The model under review builds one solid part; all positions refer to its coordinate system, in mm. A direction names the side the tool comes from. Round coordinates to 2 decimals unless told otherwise and drop trailing zeros. Order: outer loops, then holes, each group sorted by start corner. A loop starts at its lowest first (then second) coordinate and runs counter-clockwise, first axis right, second up. Notation, with made-up numbers: M -29,69.25 L 0,69.25 A13 ccw 0,76.25 Z; hole C 44,7 d4. An arc over 180 degrees is marked long. Answer as a JSON object with one key per item and string values. Group by question number.
1) Consider section D-D, the plane y = -8.25. Write out the cut boundary in (x, z), then the cut area to 3 significant figures.
2) To check wall thickness, follow line 1 (Y direction, x = 19, z = 32); line 2 (X direction, y = -21.75, z = -34.5); line 3 (Z direction, x = 38, y = -12.25). State the ranges of each line that lie inside material, in increasing order.
3) Consider section B-B, the plane y = -17. Write out the cut boundary in (x, z), then the cut area to 3 significant figures.
4) Consider section C-C, the plane z = 25.5. Write out the cut boundary in (x, y).
5) Consider section A-A, the plane x = -28.5. Write out the cut boundary in (y, z), then the cut area to 3 significant figures.
6) Insertion check: pin 1 Ø12 at (x, z) = (-23, -0.5) entering from -Y; pin 2 Ø10 at (x, z) = (-68, 15.5) entering from +Y; pin 3 Ø1.3 at (x, y) = (-32, -26.5) entering from -Z. Each pin has a flat end and moves straight along its axis. Give the tip position at first contact, or say it passes through.
7) For faces 1 (the cylindrical face through (42.55, -2.02, 8.81)), 2 (the flat face through (-30, -28, 32.298)), 3 (the cylindrical face through (-65.101, -22.062, 4.926)), 4 (the flat face through (-30, -28, 21.446)), 5 (the flat face through (-21.4, -28, 27)), list the 3-axis set-ups (+Z, -Z, +X, -X, +Y, -Y) from which the entire face can be reached by the end or side of a thin tool; tool diameter is ignored.
```python
from build123d import *

# Parameters (mm, degrees)
F0_W      = 68.2077519596
F0_H      = 90.4731266201
F1_DEPTH  = 25.4
F2_R      = 10.4447594079
F3_DEPTH  = 30.0825480372
F4_R      = 9.9602632564
F5_DEPTH  = 25.4
F6_DEPTH  = 14.6486386657
F7_DEPTH  = 77.0113542676
F8_DEPTH  = 7.2514917701
F9_DEPTH  = 2.6144357398
F10_W     = 17.0795619488
F10_H     = 10.8526591212
F11_DEPTH = 4.2919376865


with BuildPart() as f1:
    # F0 (on Front) → F1 (new body)
    with BuildSketch(Plane.XZ):
        with Locations((-11.2533476204, -0.3619696945)):
            Rectangle(F0_W, F0_H)
    extrude(amount=F1_DEPTH)

    # F2 (on face) → F3 (join)
    with BuildSketch(Plane.YZ.offset(22.8505283594)):
        with Locations((-11.9834244251, 5.6728608906)):
            Circle(F2_R)
    extrude(amount=F3_DEPTH)

    # F4 (on face) → F5 (join)
    with BuildSketch(Plane(origin=(-45.3572236001, 0, 0), x_dir=(0, -1, 0), z_dir=(-1, 0, 0))):
        with Locations((12.8610506654, 8.7403887883)):
            Circle(F4_R)
    extrude(amount=F5_DEPTH)

    # F6 (add): a face of the model
    f6_faces = [f1.faces().sort_by_distance(p)[0] for p in [
        (-70.7572236001, -12.8610506654, 8.7403887883),
    ]]
    extrude(f6_faces, amount=F6_DEPTH)

    # F7 (add): a face of the model
    f7_faces = [f1.faces().sort_by_distance(p)[0] for p in [
        (-85.4058622658, -12.8610506654, 8.7403887883),
    ]]
    extrude(f7_faces, amount=-F7_DEPTH)

    # F8 (add): a face of the model
    f8_faces = [f1.faces().sort_by_distance(p)[0] for p in [
        (52.9330763966, -11.9834244251, 5.6728608906),
    ]]
    extrude(f8_faces, amount=F8_DEPTH)

    # F9 (add): a face of the model
    f9_faces = [f1.faces().sort_by_distance(p)[0] for p in [
        (60.1845681667, -11.9834244251, 5.6728608906),
    ]]
    extrude(f9_faces, amount=F9_DEPTH)

    # F10 (on face) → F11 (join)
    with BuildSketch(Plane.XZ.offset(25.4)):
        with Locations((-29.9396589398, 26.8718404695)):
            Rectangle(F10_W, F10_H)
    extrude(amount=F11_DEPTH)


solid = f1.part
```
Results list:
{
 "1": {"outline": "M -85.41,-0.09 L -45.36,-0.09 L -45.36,-45.6 L 22.85,-45.6 L 22.85,-4.08 L 62.8,-4.08 L 62.8,15.43 L 22.85,15.43 L 22.85,44.87 L -45.36,44.87 L -45.36,17.57 L -85.41,17.57 Z", "area": "7,660 mm^2"},
 "2": {"line 1": "-25.4 to 0", "line 2": "-45.36 to 22.85", "line 3": "-4.77 to 16.11"},
 "3": {"outline": "M -85.41,-0.32 L -45.36,-0.32 L -45.36,-45.6 L 22.85,-45.6 L 22.85,-3.49 L 62.8,-3.49 L 62.8,14.83 L 22.85,14.83 L 22.85,44.87 L -45.36,44.87 L -45.36,17.8 L -85.41,17.8 Z", "area": "7,630 mm^2"},
 "4": {"outline": "M -45.36,-25.4 L -38.48,-25.4 L -38.48,-29.69 L -21.4,-29.69 L -21.4,-25.4 L 22.85,-25.4 L 22.85,0 L -45.36,0 Z"},
 "5": {"outline": "M -29.69,21.45 L -25.4,21.45 L -25.4,-45.6 L 0,-45.6 L 0,44.87 L -25.4,44.87 L -25.4,32.3 L -29.69,32.3 Z", "area": "2,340 mm^2"},
 "6": {"pin 1": "y = -25.4", "pin 2": "y = -3.06", "pin 3": "z = 21.45"},
 "7": {"face 1": "+X", "face 2": "+Z, +X, -X, -Y", "face 3": "-X", "face 4": "-Z, +X, -X, -Y", "face 5": "+Z, -Z, +X, -Y"}
}
